Geometry: see drawing. Coordinates: mm, zero at the bounding-box minimum. Coordinates: 2 decimals unless noted, no trailing zeros. Order: outer loops, then holes, each group sorted by start corner. A loop starts at its lowest first (then second) coordinate and runs counter-clockwise, first axis right, second up.
Item 1: Section C-C on y = 5.5. Return the cut outline in (x, z), then the cut area to 3 significant figures.
Item 2: Ray query, line 1 (X direction, y = 2, z = 125.5); line 2 (Z direction, x = 33, y = 5.25); line 3 (Z direction, x = 88, y = 4.25) (1 decimal). Return the intervals inside material, ascending.
Item 3: Section A-A on x = 27. Return the cut outline in (y, z).
Item 4: Section B-B on z = 80. Return the cut outline in (x, y), then the cut area to 3 significant figures.
Item 5: Contact query for a flat-ended pin moving along its axis: P1, Ø2, axis at y = 5, z = 23.5, coming from the -X side (1 decimal). Output: stop coordinate, or through.
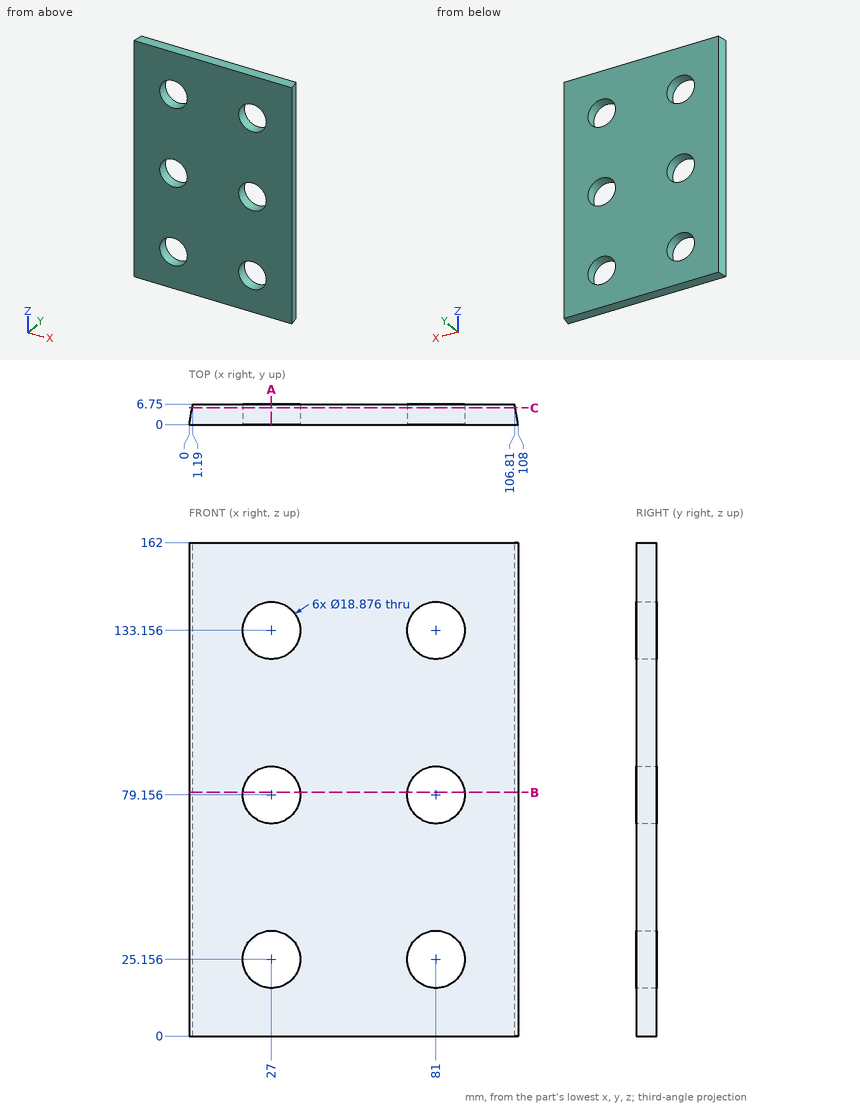
Answer list:
1. outline: (0.97, 0) - (107.03, 0) - (107.03, 162) - (0.97, 162) - close; hole circle Ø18.88 at (27, 25.16); hole circle Ø18.88 at (27, 79.16); hole circle Ø18.88 at (27, 133.16); hole circle Ø18.88 at (81, 25.16); hole circle Ø18.88 at (81, 79.16); hole circle Ø18.88 at (81, 133.16)
1. area: 15,500 mm2
2. line 1: x = 0.35 to 21.48, 32.52 to 75.48, 86.52 to 107.65
2. line 2: z = 0 to 17.87, 32.44 to 71.87, 86.44 to 125.87, 140.44 to 162
2. line 3: z = 0 to 18.8, 31.5 to 72.8, 85.5 to 126.8, 139.5 to 162
3. outline: (0, 0) - (6.75, 0) - (6.75, 15.72) - (0, 15.72) - close; (0, 34.59) - (6.75, 34.59) - (6.75, 69.72) - (0, 69.72) - close; (0, 88.59) - (6.75, 88.59) - (6.75, 123.72) - (0, 123.72) - close; (0, 142.59) - (6.75, 142.59) - (6.75, 162) - (0, 162) - close
4. outline: (0, 0) - (17.6, 0) - (17.6, 6.75) - (1.19, 6.75) - close; (36.4, 0) - (71.6, 0) - (71.6, 6.75) - (36.4, 6.75) - close; (90.4, 0) - (108, 0) - (106.81, 6.75) - (90.4, 6.75) - close
4. area: 467 mm2
5. P1: stops at x = 0.7
